Could you check a few things on this model? Use its own coordinates, in mm. Face numbers are marked on the shaded views. Give positions to 0.01 mm unless a question says otherwise; leave off trailing zeros. Order: outer loops, then holes, each group sorted by start corner. A loop starts at its lowest first (then second) coordinate and runs counter-clockwise, first axis right, second up. Notation, with made-up numbers: M 27.25,73.25 L 66.25,73.25 A22 ccw 66.25,79.25 Z; hole C -6,56 d2. An arc over 180 degrees is marked long. Use a Markdown table: item, result. Add a question column.
Item 1: Suppose I cut it at D-D on y = 1.3. Count the separate pieces of the cut face and the enclosed holes in it, plus the area to 3 significant figures.
Item 2: If I drill on L1, parallel to X at y = 3.35, z = 14.5; L2, parallel to X at y = 1.9, z = 67; L3, parallel to Z at x = -31.5, y = 3.6, over which ranges is the centre line in solid material (lowest first)? Write a range as from..to.
Item 3: I'm going to push a flat-ended pin straight in: pin 1 Ø2.5 at (y, z) = (3.5, 28.5) entering from -X. Where does the tip first touch, or does it pass through?
Item 4: Suppose I cut it at A-A on x = -62.5. Write out the boundary of the cut face in (y, z).
Item 5: If we mould it in two halves opening along X, with no side actions, what happens to the marked faces 1 and 2? For each: released by +X, released by -X, zero draft, split by the parting line, or undercut.
Item 6: Suppose I cut it at C-C on x = -16. Write out the boundary of the cut face in (y, z).
Item 7: Suppose I cut it at B-B on z = -28.5. Write out the boundary of the cut face in (x, y), plus the area to 3 significant figures.
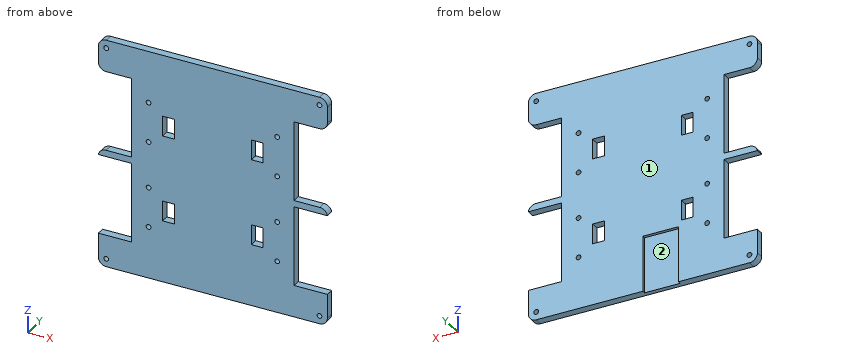
from build123d import *

# Parameters (mm, degrees)
SKETCH1_W           = 144
SKETCH1_H           = 144
BOSS_EXTRUDE1_DEPTH = 5
SKETCH2_W           = 21
SKETCH2_H           = 50
CUT_EXTRUDE1_DEPTH  = 5
SKETCH11_W          = 7.4
SKETCH11_H          = 12.6
CUT_EXTRUDE10_DEPTH = 5
SKETCH13_R          = 1.5
CUT_EXTRUDE12_DEPTH = 5
FILLET1_R           = 5
FILLET2_R           = 5
FILLET3_R           = 5
SKETCH14_R          = 1.5
CUT_EXTRUDE13_DEPTH = 5
SKETCH15_W          = 22.44
SKETCH15_H          = 35
CUT_EXTRUDE14_DEPTH = 2


with BuildPart() as part:
    # Sketch1 → Boss-Extrude1 (new body)
    with BuildSketch(Plane(origin=(0, 0, 0), x_dir=(1, 0, 0), z_dir=(0, 1, 0))):
        Rectangle(SKETCH1_W, SKETCH1_H)
    extrude(amount=BOSS_EXTRUDE1_DEPTH)

    # Sketch2 → Cut-Extrude1 (cut)
    with BuildSketch(Plane(origin=(0, 5, 0), x_dir=(1, 0, 0), z_dir=(0, 1, 0))):
        with Locations((-61.5, -27)):
            Rectangle(SKETCH2_W, SKETCH2_H)
        with Locations((61.5, -27)):
            Rectangle(SKETCH2_W, SKETCH2_H)
        with Locations((61.5, 27)):
            Rectangle(SKETCH2_W, SKETCH2_H)
        with Locations((-61.5, 27)):
            Rectangle(SKETCH2_W, SKETCH2_H)
    extrude(amount=-CUT_EXTRUDE1_DEPTH, mode=Mode.SUBTRACT)

    # Sketch11 → Cut-Extrude10 (cut)
    with BuildSketch(Plane(origin=(0, 5, 0), x_dir=(1, 0, 0), z_dir=(0, 1, 0))):
        with Locations((27.945388191, -26.98248673)):
            Rectangle(SKETCH11_W, SKETCH11_H)
        with Locations((-27.945388191, -26.98248673)):
            Rectangle(SKETCH11_W, SKETCH11_H)
        with Locations((27.945388191, 26.98248673)):
            Rectangle(SKETCH11_W, SKETCH11_H)
        with Locations((-27.945388191, 26.98248673)):
            Rectangle(SKETCH11_W, SKETCH11_H)
    extrude(amount=-CUT_EXTRUDE10_DEPTH, mode=Mode.SUBTRACT)

    # Sketch13 → Cut-Extrude12 (cut)
    with BuildSketch(Plane(origin=(0, 5, 0), x_dir=(1, 0, 0), z_dir=(0, 1, 0))):
        with Locations(Location((-67, 67, 0), (0, 0, 270))):
            Circle(SKETCH13_R)
        with Locations(Location((-67, -67, 0), (0, 0, 270))):
            Circle(SKETCH13_R)
        with Locations(Location((67, 67, 0), (0, 0, 270))):
            Circle(SKETCH13_R)
        with Locations(Location((67, -67, 0), (0, 0, 270))):
            Circle(SKETCH13_R)
    extrude(amount=-CUT_EXTRUDE12_DEPTH, mode=Mode.SUBTRACT)

    # Fillet1
    fillet1_edges = [part.edges().sort_by_distance(p)[0] for p in [
        (-72, 2.5, -72),
    ]]
    fillet(fillet1_edges, radius=FILLET1_R)

    # Fillet2
    # the kernel refuses this fillet: 5 mm, written as the material it takes off along each edge
    with BuildSketch(Plane(origin=(-72, 17.5, 52), x_dir=(1, 0, 0), z_dir=(0, -1, 0))) as fillet2_piece_1:
        with BuildLine():
            CenterArc((FILLET2_R, FILLET2_R), FILLET2_R, 180, 90)
            Line((0, FILLET2_R), (-FILLET2_R * 0.02, FILLET2_R))
            Line((-FILLET2_R * 0.02, FILLET2_R), (-FILLET2_R * 0.02, -FILLET2_R * 0.02))
            Line((-FILLET2_R * 0.02, -FILLET2_R * 0.02), (FILLET2_R, -FILLET2_R * 0.02))
            Line((FILLET2_R, -FILLET2_R * 0.02), (FILLET2_R, 0))
        make_face()
    extrude(amount=30, mode=Mode.SUBTRACT)
    with BuildSketch(Plane(origin=(-72, 17.247448714, 2), x_dir=(1.5631940186717212e-12, 0, -1.0), z_dir=(0, -1, 0))) as fillet2_piece_2:
        with BuildLine():
            CenterArc((5, 4.898979486), FILLET2_R, 180, 78.463040967)
            Line((0, 4.898979486), (-0.1, 4.898979486))
            Line((-0.1, 4.898979486), (-0.1, 0))
            Line((-0.1, 0), (0, -0.1))
            ThreePointArc((0, -0.1), (2, -0.1), (3.98, -0.09797959))
            Line((3.98, -0.09797959), (4, 0))
        make_face()
    extrude(amount=29.494897428, mode=Mode.SUBTRACT)
    with BuildSketch(Plane(origin=(-72, -12.5, 72), x_dir=(0, 0, -1), z_dir=(0, 1, 0))) as fillet2_piece_3:
        with BuildLine():
            CenterArc((FILLET2_R, -FILLET2_R), FILLET2_R, 90, 90)
            Line((0, -FILLET2_R), (-FILLET2_R * 0.02, -FILLET2_R))
            Line((-FILLET2_R * 0.02, -FILLET2_R), (-FILLET2_R * 0.02, FILLET2_R * 0.02))
            Line((-FILLET2_R * 0.02, FILLET2_R * 0.02), (FILLET2_R, FILLET2_R * 0.02))
            Line((FILLET2_R, FILLET2_R * 0.02), (FILLET2_R, 0))
        make_face()
    extrude(amount=30, mode=Mode.SUBTRACT)

    # Fillet3
    # the kernel refuses this fillet: 5 mm, written as the material it takes off along each edge
    with BuildSketch(Plane(origin=(72, 17.247448714, 2), x_dir=(-1, 0, 0), z_dir=(0, -1, 0))) as fillet3_piece_1:
        with BuildLine():
            CenterArc((4.898979486, 5), FILLET3_R, 191.536959033, 78.463040967)
            Line((0, 4), (-0.09797959, 3.98))
            ThreePointArc((-0.09797959, 3.98), (-0.1, 2), (-0.1, 0))
            Line((-0.1, 0), (0, -0.1))
            Line((0, -0.1), (4.898979486, -0.1))
            Line((4.898979486, -0.1), (4.898979486, 0))
        make_face()
    extrude(amount=29.494897428, mode=Mode.SUBTRACT)
    with BuildSketch(Plane(origin=(72, 17.5, 52), x_dir=(0, 0, 1), z_dir=(0, -1, 0)), Plane(origin=(72, -12.5, -72), x_dir=(-1, 0, 0), z_dir=(0, 1, 0))) as fillet3_piece_2:
        with BuildLine():
            CenterArc((FILLET3_R, FILLET3_R), FILLET3_R, 180, 90)
            Line((0, FILLET3_R), (-FILLET3_R * 0.02, FILLET3_R))
            Line((-FILLET3_R * 0.02, FILLET3_R), (-FILLET3_R * 0.02, -FILLET3_R * 0.02))
            Line((-FILLET3_R * 0.02, -FILLET3_R * 0.02), (FILLET3_R, -FILLET3_R * 0.02))
            Line((FILLET3_R, -FILLET3_R * 0.02), (FILLET3_R, 0))
        make_face()
    extrude(amount=30, mode=Mode.SUBTRACT)
    with BuildSketch(Plane(origin=(72, -12.5, 72), x_dir=(-1, 0, 0), z_dir=(0, 1, 0))) as fillet3_piece_3:
        with BuildLine():
            CenterArc((FILLET3_R, -FILLET3_R), FILLET3_R, 90, 90)
            Line((0, -FILLET3_R), (-FILLET3_R * 0.02, -FILLET3_R))
            Line((-FILLET3_R * 0.02, -FILLET3_R), (-FILLET3_R * 0.02, FILLET3_R * 0.02))
            Line((-FILLET3_R * 0.02, FILLET3_R * 0.02), (FILLET3_R, FILLET3_R * 0.02))
            Line((FILLET3_R, FILLET3_R * 0.02), (FILLET3_R, 0))
        make_face()
    extrude(amount=30, mode=Mode.SUBTRACT)

    # Sketch14 → Cut-Extrude13 (cut)
    with BuildSketch(Plane.XZ):
        with Locations(Location((-40.4, 39.5, 0), (0, 0, 270))):
            Circle(SKETCH14_R)
        with Locations(Location((-40.4, 14.5, 0), (0, 0, 270))):
            Circle(SKETCH14_R)
        with Locations(Location((40.4, 39.5, 0), (0, 0, 270))):
            Circle(SKETCH14_R)
        with Locations(Location((40.4, 14.5, 0), (0, 0, 270))):
            Circle(SKETCH14_R)
        with Locations(Location((-40.4, -14.5, 0), (0, 0, 270))):
            Circle(SKETCH14_R)
        with Locations(Location((-40.4, -39.5, 0), (0, 0, 270))):
            Circle(SKETCH14_R)
        with Locations(Location((40.4, -14.5, 0), (0, 0, 270))):
            Circle(SKETCH14_R)
        with Locations(Location((40.4, -39.5, 0), (0, 0, 270))):
            Circle(SKETCH14_R)
    extrude(amount=-CUT_EXTRUDE13_DEPTH, mode=Mode.SUBTRACT)

    # Sketch15 → Cut-Extrude14 (cut)
    with BuildSketch(Plane(origin=(0, 5, 0), x_dir=(1, 0, 0), z_dir=(0, 1, 0))):
        with Locations((-11.22, 54.5)):
            Rectangle(SKETCH15_W, SKETCH15_H)
    extrude(amount=-CUT_EXTRUDE14_DEPTH, mode=Mode.SUBTRACT)


solid = part.part
Findings below:
| question | item | result |
|---|---|---|
| 1 | separate pieces | 1 |
| 1 | enclosed holes | 16 |
| 1 | area | 16,000 mm^2 |
| 2 | L1 | x = -51..-41.9, -38.9..38.9, 41.9..51 |
| 2 | L2 | x = -72..-68.5, -65.5..65.5, 68.5..72 |
| 2 | L3 | z = -72..-33.28, -20.68..20.68, 33.28..72 |
| 3 | pin 1 | stops at x = -51 |
| 4 | outline | M 0,-72 L 5,-72 L 5,-52 L 0,-52 Z; M 0,-2 L 5,-2 L 5,2 L 0,2 Z; M 0,52 L 5,52 L 5,72 L 0,72 Z |
| 5 | face 1 | zero draft |
| 5 | face 2 | undercut |
| 6 | outline | M 0,-72 L 3,-72 L 3,-37 L 5,-37 L 5,72 L 0,72 Z |
| 7 | outline | M -51,0 L -31.65,0 L -31.65,5 L -51,5 Z; M -24.25,0 L 24.25,0 L 24.25,5 L -24.25,5 Z; M 31.65,0 L 51,0 L 51,5 L 31.65,5 Z |
| 7 | area | 436 mm^2 |
